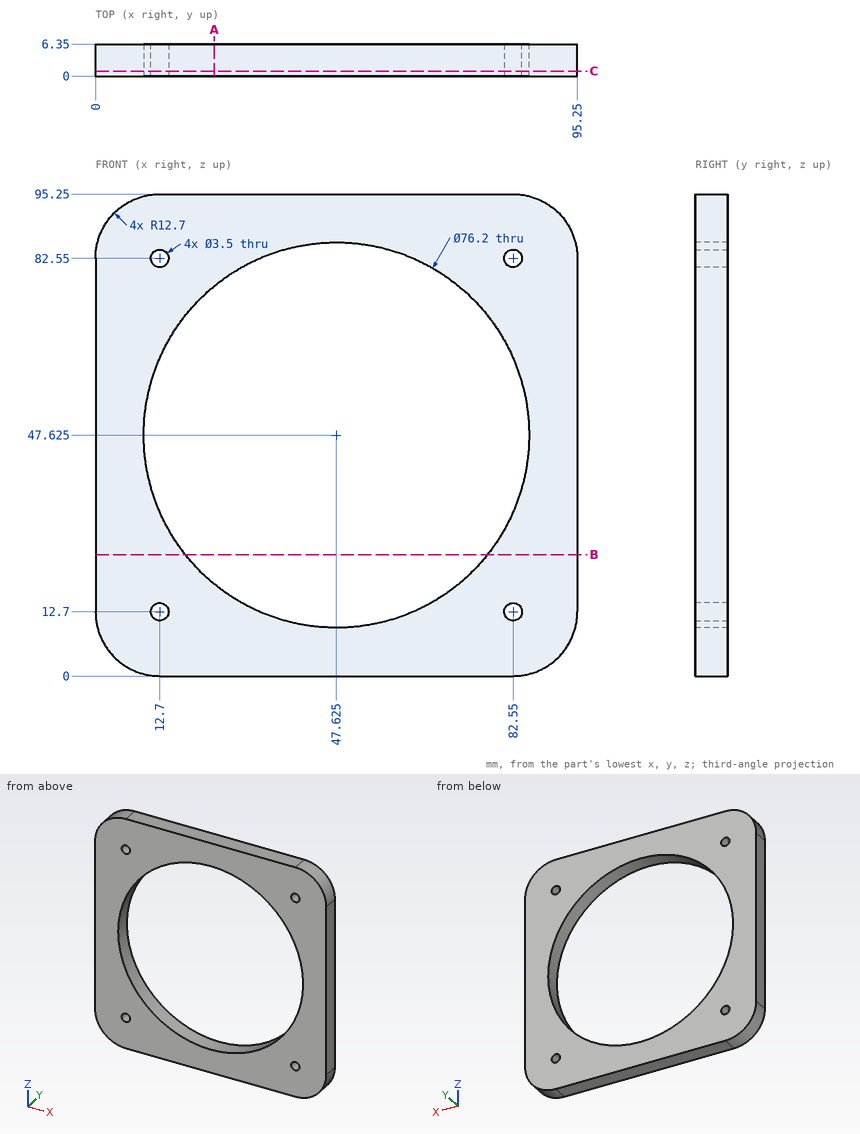
Study the drawing (mm; zero at the part's minimum x, y, z) and answer. Give positions to 0.01 mm unless a question says otherwise; leave off trailing zeros. Write each loop counter-clockwise with the first axis right and the second up, starting at its lowest first coordinate (ties: lowest second). Pieces come first, ordered by that corner, then holes. Notation, with made-up numbers: (54.5, 29) - (58.5, 29) arc R17 cw to (58.5, 38) - close; hole circle Ø2 at (68, -15.5). An arc over 180 degrees is marked (long way). One line per question, with ' | ' between items. Start each with the question number.
1. Section A-A, the plane x = 23.5 is taken. Determine the outline of the cut face in (y, z).
2. Straight lines are drawn through the part: line 1 (X direction, y = 4, z = 47); line 2 (Z direction, x = 12.7, y = 4.75); line 3 (Z direction, x = 77, y = 4.75). For each, find the intervals that lie inside material, in ascending order.
3. Section B-B, the plane z = 24 is taken. Determine the outline of the cut face in (x, y), then the cut area to 3 significant figures.
4. Section C-C, the plane y = 1 is taken. Determine the outline of the cut face in (x, z) (3 decimals).
Result:
1) outline: (0, 0) - (6.35, 0) - (6.35, 18.14) - (0, 18.14) - close; (0, 77.11) - (6.35, 77.11) - (6.35, 95.25) - (0, 95.25) - close
2) line 1: x = 0 to 9.53, 85.72 to 95.25 | line 2: z = 0 to 10.95, 14.45 to 32.4, 62.85 to 80.8, 84.3 to 95.25 | line 3: z = 0 to 23.36, 71.89 to 95.25
3) outline: (0, 0) - (17.73, 0) - (17.73, 6.35) - (0, 6.35) - close; (77.52, 0) - (95.25, 0) - (95.25, 6.35) - (77.52, 6.35) - close | area: 225 mm2
4) outline: (0, 12.7) arc R12.7 ccw to (12.7, 0) - (82.55, 0) arc R12.7 ccw to (95.25, 12.7) - (95.25, 82.55) arc R12.7 ccw to (82.55, 95.25) - (12.7, 95.25) arc R12.7 ccw to (0, 82.55) - close; hole circle Ø76.2 at (47.625, 47.625); hole circle Ø3.5 at (12.7, 12.7); hole circle Ø3.5 at (12.7, 82.55); hole circle Ø3.5 at (82.55, 12.7); hole circle Ø3.5 at (82.55, 82.55)
